from build123d import *

# Parameters (mm, degrees)
SKETCH_1_R      = 1.5
SKETCH_1_R_2    = 3
SKETCH_1_W      = 52
SKETCH_1_H      = 52
EXTRUDE_1_DEPTH = 3


with BuildPart() as part:
    # 草图1 → 凸台-拉伸1 (new body)
    with BuildSketch(Plane(origin=(0, 0, 0), x_dir=(1, 0, 0), z_dir=(0, 1, 0))):
        Polygon((-140, -50), (-70, -50), (-70, 25), (70, 25), (70, -50), (140, -50), (140, 95), (-140, 95), align=None)
        with Locations(Location((0, 80, 0), (0, 0, 270))):
            Circle(SKETCH_1_R, mode=Mode.SUBTRACT)
        with Locations(Location((0, 35, 0), (0, 0, 270))):
            Circle(SKETCH_1_R, mode=Mode.SUBTRACT)
        with Locations(Location((0, 70, 0), (0, 0, 270))):
            Circle(SKETCH_1_R_2, mode=Mode.SUBTRACT)
        with Locations((36, 59)):
            Rectangle(SKETCH_1_W, SKETCH_1_H, mode=Mode.SUBTRACT)
        with Locations((-36, 59)):
            Rectangle(SKETCH_1_W, SKETCH_1_H, mode=Mode.SUBTRACT)
        with Locations((-108, 59)):
            Rectangle(SKETCH_1_W, SKETCH_1_H, mode=Mode.SUBTRACT)
        with Locations((108, 59)):
            Rectangle(SKETCH_1_W, SKETCH_1_H, mode=Mode.SUBTRACT)
        with Locations((-108, -13)):
            Rectangle(SKETCH_1_W, SKETCH_1_H, mode=Mode.SUBTRACT)
        with Locations((108, -13)):
            Rectangle(SKETCH_1_W, SKETCH_1_H, mode=Mode.SUBTRACT)
    extrude(amount=EXTRUDE_1_DEPTH)


solid = part.part
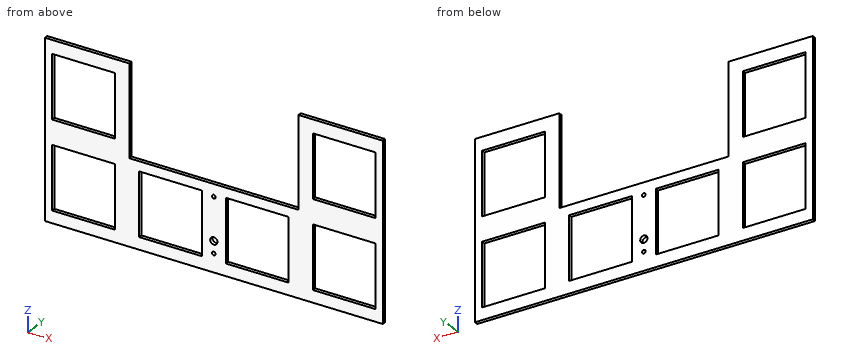
The listing builds one solid part. Answer for the finished solid, in the listing's coordinates (mm). Round coordinates to 2 decimals unless told otherwise and drop trailing zeros. Write each loop counter-clockwise with the first axis right and the second up, starting at its lowest first coordinate (ties: lowest second). Pieces come first, ordered by that corner, then holes. Notation, with made-up numbers: (54.5, 52.25) - (70.5, 52.25) arc R32 ccw to (70.5, 83.25) - close; hole circle Ø7 at (53.25, 7). An arc over 180 degrees is marked (long way). Use a Markdown table: item, result. Add a question column.
1. The part is cut by section C-C (z = -70). Write down the section's boundary in (x, y), and give its area (3 significant figures).
2. Consider line 1 (X direction, y = 2.85, z = 15); line 2 (X direction, y = 1.55, z = -35); line 3 (X direction, y = 0.9, z = -45.5). Determine where each line is inside the solid, lowest interval first.
3. The part is cut by section B-B (x = -97). Write down the section's boundary in (y, z), and give its area (3 significant figures).
4. The part is cut by section A-A (z = 31). Write down the section's boundary in (x, y).
5. The part is cut by section D-D (x = 48.5). Write down the section's boundary in (y, z).
Reported:
| question | item | result |
|---|---|---|
| 1 | outline | (-140, 0) - (-134, 0) - (-134, 3) - (-140, 3) - close; (-82, 0) - (-62, 0) - (-62, 3) - (-82, 3) - close; (-10, 0) - (-3, 0) - (-3, 3) - (-10, 3) - close; (3, 0) - (10, 0) - (10, 3) - (3, 3) - close; (62, 0) - (82, 0) - (82, 3) - (62, 3) - close; (134, 0) - (140, 0) - (140, 3) - (134, 3) - close |
| 1 | area | 198 mm^2 |
| 2 | line 1 | -140 to -134, -82 to -70, 70 to 82, 134 to 140 |
| 2 | line 2 | -140 to -134, -82 to -62, -10 to -1.5, 1.5 to 10, 62 to 82, 134 to 140 |
| 2 | line 3 | -140 to -134, -82 to -62, -10 to 10, 62 to 82, 134 to 140 |
| 3 | outline | (0, -95) - (3, -95) - (3, -85) - (0, -85) - close; (0, -33) - (3, -33) - (3, -13) - (0, -13) - close; (0, 39) - (3, 39) - (3, 50) - (0, 50) - close |
| 3 | area | 123 mm^2 |
| 4 | outline | (-140, 0) - (-134, 0) - (-134, 3) - (-140, 3) - close; (-82, 0) - (-70, 0) - (-70, 3) - (-82, 3) - close; (70, 0) - (82, 0) - (82, 3) - (70, 3) - close; (134, 0) - (140, 0) - (140, 3) - (134, 3) - close |
| 5 | outline | (0, -95) - (3, -95) - (3, -85) - (0, -85) - close; (0, -33) - (3, -33) - (3, -25) - (0, -25) - close |
